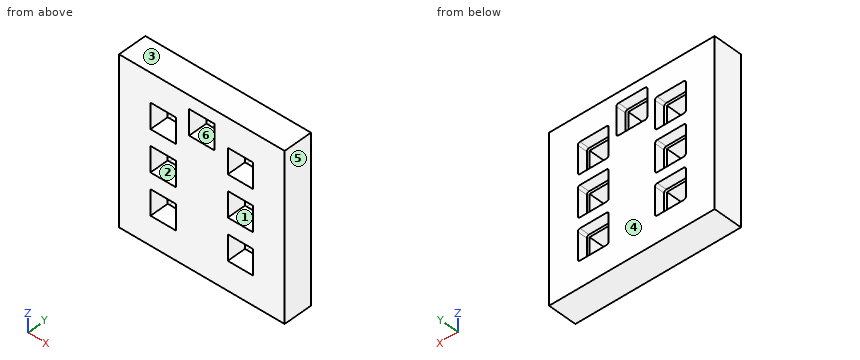
from build123d import *

# Parameters (mm, degrees)
SKETCH1_W           = 150
SKETCH1_H           = 150
BOSS_EXTRUDE1_DEPTH = 26
CUT_EXTRUDE1_DEPTH  = 9
SKETCH3_W           = 23
SKETCH3_H           = 23
CUT_EXTRUDE2_DEPTH  = 18


with BuildPart() as part:
    # Sketch1 → Boss-Extrude1 (new body)
    with BuildSketch(Plane(origin=(0, 0, 0), x_dir=(1, 0, 0), z_dir=(0, 1, 0))):
        Rectangle(SKETCH1_W, SKETCH1_H)
    extrude(amount=BOSS_EXTRUDE1_DEPTH)

    # Sketch2 → Cut-Extrude1 (cut)
    with BuildSketch(Plane(origin=(0, 26, 0), x_dir=(1, 0, 0), z_dir=(0, 1, 0))):
        with BuildLine():
            Line((-47, 23.5), (-23, 23.5))
            ThreePointArc((-23, 23.5), (-21.585786438, 24.085786438), (-21, 25.5))
            Line((-21, 25.5), (-21, 49.5))
            ThreePointArc((-21, 49.5), (-21.585786438, 50.914213562), (-23, 51.5))
            Line((-23, 51.5), (-47, 51.5))
            ThreePointArc((-47, 51.5), (-48.414213562, 50.914213562), (-49, 49.5))
            Line((-49, 49.5), (-49, 25.5))
            ThreePointArc((-49, 25.5), (-48.414213562, 24.085786438), (-47, 23.5))
        make_face()
        with BuildLine():
            Line((-47, 14), (-23, 14))
            ThreePointArc((-23, 14), (-21.585786438, 13.414213562), (-21, 12))
            Line((-21, 12), (-21, -12))
            ThreePointArc((-21, -12), (-21.585786438, -13.414213562), (-23, -14))
            Line((-23, -14), (-47, -14))
            ThreePointArc((-47, -14), (-48.414213562, -13.414213562), (-49, -12))
            Line((-49, -12), (-49, 12))
            ThreePointArc((-49, 12), (-48.414213562, 13.414213562), (-47, 14))
        make_face()
        with BuildLine():
            Line((-21, -49.5), (-21, -25.5))
            ThreePointArc((-21, -25.5), (-21.585786438, -24.085786438), (-23, -23.5))
            Line((-23, -23.5), (-47, -23.5))
            ThreePointArc((-47, -23.5), (-48.414213562, -24.085786438), (-49, -25.5))
            Line((-49, -25.5), (-49, -49.5))
            ThreePointArc((-49, -49.5), (-48.414213562, -50.914213562), (-47, -51.5))
            Line((-47, -51.5), (-23, -51.5))
            ThreePointArc((-23, -51.5), (-21.585786438, -50.914213562), (-21, -49.5))
        make_face()
        with BuildLine():
            Line((47, -23.5), (23, -23.5))
            ThreePointArc((23, -23.5), (21.585786438, -24.085786438), (21, -25.5))
            Line((21, -25.5), (21, -49.5))
            ThreePointArc((21, -49.5), (21.585786438, -50.914213562), (23, -51.5))
            Line((23, -51.5), (47, -51.5))
            ThreePointArc((47, -51.5), (48.414213562, -50.914213562), (49, -49.5))
            Line((49, -49.5), (49, -25.5))
            ThreePointArc((49, -25.5), (48.414213562, -24.085786438), (47, -23.5))
        make_face()
        with BuildLine():
            Line((21, 49.5), (21, 25.5))
            ThreePointArc((21, 25.5), (21.585786438, 24.085786438), (23, 23.5))
            Line((23, 23.5), (47, 23.5))
            ThreePointArc((47, 23.5), (48.414213562, 24.085786438), (49, 25.5))
            Line((49, 25.5), (49, 49.5))
            ThreePointArc((49, 49.5), (48.414213562, 50.914213562), (47, 51.5))
            Line((47, 51.5), (23, 51.5))
            ThreePointArc((23, 51.5), (21.585786438, 50.914213562), (21, 49.5))
        make_face()
        with BuildLine():
            Line((21, 12), (21, -12))
            ThreePointArc((21, -12), (21.585786438, -13.414213562), (23, -14))
            Line((23, -14), (47, -14))
            ThreePointArc((47, -14), (48.414213562, -13.414213562), (49, -12))
            Line((49, -12), (49, 12))
            ThreePointArc((49, 12), (48.414213562, 13.414213562), (47, 14))
            Line((47, 14), (23, 14))
            ThreePointArc((23, 14), (21.585786438, 13.414213562), (21, 12))
        make_face()
        with BuildLine():
            Line((-12, -37.5), (12, -37.5))
            ThreePointArc((12, -37.5), (13.414213562, -38.085786438), (14, -39.5))
            Line((14, -39.5), (14, -63.5))
            ThreePointArc((14, -63.5), (13.414213562, -64.914213562), (12, -65.5))
            Line((12, -65.5), (-12, -65.5))
            ThreePointArc((-12, -65.5), (-13.414213562, -64.914213562), (-14, -63.5))
            Line((-14, -63.5), (-14, -39.5))
            ThreePointArc((-14, -39.5), (-13.414213562, -38.085786438), (-12, -37.5))
        make_face()
    extrude(amount=-CUT_EXTRUDE1_DEPTH, mode=Mode.SUBTRACT)

    # Sketch3 → Cut-Extrude2 (cut, through all)
    with BuildSketch(Plane(origin=(0, 17, 0), x_dir=(1, 0, 0), z_dir=(0, 1, 0))):
        with Locations((-35, -37.5)):
            Rectangle(SKETCH3_W, SKETCH3_H)
        with Locations((-35, 37.5)):
            Rectangle(SKETCH3_W, SKETCH3_H)
        with Locations((35, -37.5)):
            Rectangle(SKETCH3_W, SKETCH3_H)
        with Locations((35, 37.5)):
            Rectangle(SKETCH3_W, SKETCH3_H)
        with Locations((-35, 0)):
            Rectangle(SKETCH3_W, SKETCH3_H)
        with Locations((35, 0)):
            Rectangle(SKETCH3_W, SKETCH3_H)
        with Locations((0, -51.5)):
            Rectangle(SKETCH3_W, SKETCH3_H)
    extrude(amount=-CUT_EXTRUDE2_DEPTH, mode=Mode.SUBTRACT)


solid = part.part
Read the model definition and answer for the solid it produces. Units are mm, in the model's axes. Face numbers are marked on the shaded views. A direction names the side the tool comes from. Coordinates: 2 decimals unless noted, no trailing zeros. Write each loop counter-clockwise with the first axis right and the second up, starting at its lowest first coordinate (ties: lowest second). Pieces come first, ordered by that corner, then holes. Notation, with made-up numbers: M 89.5,3 L 99.5,3 A13 ccw 99.5,11 Z; hole C 46.5,7 d8. An arc over 180 degrees is marked long. Use a Markdown table: item, result.
Q1. The part is cut by section C-C, the plane y = 5.25. Give the number of separate pieces and of enclosed holes in the cut face, then the cut area to 3 significant figures.
Answer block:
| item | result |
|---|---|
| separate pieces | 1 |
| enclosed holes | 7 |
| area | 18,800 mm2 |
Q2. The part is cut by section D-D, the plane z = 33. Write down the section's boundary in (x, y).
Answer block:
| item | result |
|---|---|
| outline | M -75,0 L -46.5,0 L -46.5,17 L -49,17 L -49,26 L -75,26 Z; M -23.5,0 L 23.5,0 L 23.5,17 L 21,17 L 21,26 L -21,26 L -21,17 L -23.5,17 Z; M 46.5,0 L 75,0 L 75,26 L 49,26 L 49,17 L 46.5,17 Z |
Q3. Which of the six approach directions +Z, -Z, +X, -X, +Y, -Y give full straight-line access (tool end or side, diameter ignored) to the marked faces 5 and 6?
Answer block:
| item | result |
|---|---|
| face 5 | +Z, -Z, +X, +Y, -Y |
| face 6 | +Y, -Y |
Q4. The part is cut by section B-B, the plane z = 54. Write down the section's boundary in (x, y).
Answer block:
| item | result |
|---|---|
| outline | M -75,0 L -11.5,0 L -11.5,17 L -14,17 L -14,26 L -75,26 Z; M 11.5,0 L 75,0 L 75,26 L 14,26 L 14,17 L 11.5,17 Z |
Q5. Straight lines are drawn through the part: L1, parallel to X at y = 7, z = -42.5; L2, parallel to Z at x = 29, y = 4.75; L3, parallel to Z at x = -25.5, y = 19.5. For each, find the intervals that lie inside material, in ascending order. Write a range as [from, to].
Answer block:
| item | result |
|---|---|
| L1 | x = [-75, -46.5], [-23.5, 23.5], [46.5, 75] |
| L2 | z = [-75, -49], [-26, -11.5], [11.5, 26], [49, 75] |
| L3 | z = [-75, -51.5], [-23.5, -14], [14, 23.5], [51.5, 75] |
Q6. Determine the mould class of the marked faces 1, 2, 3 and 4 for opening direction Z: released by +Z, released by -Z, zero draft, split by the parting line, or undercut.
Answer block:
| item | result |
|---|---|
| face 1 | undercut |
| face 2 | undercut |
| face 3 | released by +Z |
| face 4 | zero draft |
Q7. The part is cut by section A-A, the plane x = 34.5. Write down the section's boundary in (y, z), then the cut area to 3 significant figures.
Answer block:
| item | result |
|---|---|
| outline | M 0,-75 L 26,-75 L 26,-51.5 L 17,-51.5 L 17,-49 L 0,-49 Z; M 0,-26 L 17,-26 L 17,-23.5 L 26,-23.5 L 26,-14 L 17,-14 L 17,-11.5 L 0,-11.5 Z; M 0,11.5 L 17,11.5 L 17,14 L 26,14 L 26,23.5 L 17,23.5 L 17,26 L 0,26 Z; M 0,49 L 17,49 L 17,51.5 L 26,51.5 L 26,75 L 0,75 Z |
| area | 1,970 mm2 |
